```python
from build123d import *

# Parameters (mm, degrees)
SKETCH1_W           = 70
SKETCH1_H           = 70
BOSS_EXTRUDE1_DEPTH = 6
SKETCH2_R           = 20
BOSS_EXTRUDE6_DEPTH = 2.6
CUT_EXTRUDE1_START  = -2.6
CUT_EXTRUDE1_DEPTH  = 2.6
SKETCH4_R           = 3.5
CUT_EXTRUDE2_DEPTH  = 1.6
SKETCH5_R           = 1
CUT_EXTRUDE3_DEPTH  = 4.4
BOSS_EXTRUDE7_DEPTH = 2


with BuildPart() as part:
    # Sketch1 → Boss-Extrude1 (new body)
    with BuildSketch(Plane(origin=(0, 0, 0), x_dir=(1, 0, 0), z_dir=(0, 1, 0))):
        Rectangle(SKETCH1_W, SKETCH1_H)
    extrude(amount=BOSS_EXTRUDE1_DEPTH)

    # Sketch2 → Boss-Extrude6 (add)
    with BuildSketch(Plane(origin=(0, 6, 0), x_dir=(1, 0, 0), z_dir=(0, 1, 0))):
        with Locations(Location((0, 0, 0), (0, 0, 270))):
            Circle(SKETCH2_R)
        with BuildLine():
            Line((-16.28125, -2.484129312), (-0.48375, -4.272702416))
            ThreePointArc((-0.48375, -4.272702416), (0, -4.3), (0.48375, -4.272702416))
            Line((0.48375, -4.272702416), (16.28125, -2.484129312))
            ThreePointArc((16.28125, -2.484129312), (18.5, 0), (16.28125, 2.484129312))
            Line((16.28125, 2.484129312), (0.48375, 4.272702416))
            ThreePointArc((0.48375, 4.272702416), (0, 4.3), (-0.48375, 4.272702416))
            Line((-0.48375, 4.272702416), (-16.28125, 2.484129312))
            ThreePointArc((-16.28125, 2.484129312), (-18.5, 0), (-16.28125, -2.484129312))
        make_face(mode=Mode.SUBTRACT)
    extrude(amount=BOSS_EXTRUDE6_DEPTH)

    # Sketch3 → Cut-Extrude1 (cut)
    with BuildSketch(Plane(origin=(0, 6, 0), x_dir=(1, 0, 0), z_dir=(0, 1, 0)).offset(CUT_EXTRUDE1_START)):
        with BuildLine():
            Line((-4.8, 3.784022013), (-4.8, -3.784022013))
            Line((-4.8, -3.784022013), (-0.48375, -4.272702416))
            ThreePointArc((-0.48375, -4.272702416), (0, -4.3), (0.48375, -4.272702416))
            Line((0.48375, -4.272702416), (4.8, -3.784022013))
            Line((4.8, -3.784022013), (4.8, 3.784022013))
            Line((4.8, 3.784022013), (0.48375, 4.272702416))
            ThreePointArc((0.48375, 4.272702416), (0, 4.3), (-0.48375, 4.272702416))
            Line((-0.48375, 4.272702416), (-4.8, 3.784022013))
        make_face()
    extrude(amount=CUT_EXTRUDE1_DEPTH, mode=Mode.SUBTRACT)

    # Sketch4 → Cut-Extrude2 (cut)
    with BuildSketch(Plane.XZ):
        with Locations(Location((16, 0, 0), (0, 0, 90))):
            Circle(SKETCH4_R)
        with Locations(Location((-16, 0, 0), (0, 0, 270))):
            Circle(SKETCH4_R)
    extrude(amount=-CUT_EXTRUDE2_DEPTH, mode=Mode.SUBTRACT)

    # Sketch5 → Cut-Extrude3 (cut)
    with BuildSketch(Plane(origin=(0, 6, 0), x_dir=(1, 0, 0), z_dir=(0, 1, 0))):
        with Locations(Location((16, 0, 0), (0, 0, 270))):
            Circle(SKETCH5_R)
        with Locations(Location((-16, 0, 0), (0, 0, 90))):
            Circle(SKETCH5_R)
    extrude(amount=-CUT_EXTRUDE3_DEPTH, mode=Mode.SUBTRACT)

    # Sketch6 → Boss-Extrude7 (add)
    with BuildSketch(Plane(origin=(0, 8.6, 0), x_dir=(1, 0, 0), z_dir=(0, 1, 0))):
        with BuildLine():
            Line((7.187033827, 3.513765042), (0.48375, 4.272702416))
            ThreePointArc((0.48375, 4.272702416), (0, 4.3), (-0.48375, 4.272702416))
            Line((-0.48375, 4.272702416), (-7.187033827, 3.513765042))
            ThreePointArc((-7.187033827, 3.513765042), (0, 8), (7.187033827, 3.513765042))
        make_face()
        with BuildLine():
            Line((0.48375, -4.272702416), (7.187033827, -3.513765042))
            ThreePointArc((7.187033827, -3.513765042), (0, -8), (-7.187033827, -3.513765042))
            Line((-7.187033827, -3.513765042), (-0.48375, -4.272702416))
            ThreePointArc((-0.48375, -4.272702416), (0, -4.3), (0.48375, -4.272702416))
        make_face()
    extrude(amount=BOSS_EXTRUDE7_DEPTH)


solid = part.part
```
Could you check a few things on this model? Use its own coordinates, in mm. A direction names the side the tool comes from. Round coordinates to 2 decimals unless told otherwise and drop trailing zeros. Write each loop counter-clockwise with the first axis right and the second up, starting at its lowest first coordinate (ties: lowest second). Pieces come first, ordered by that corner, then holes. Notation, with made-up numbers: M 0.5,-11 L 55.5,-11 A15 cw 55.5,1 Z; hole C 78,74 d8. An arc over 180 degrees is marked long. Write each question's results on one line, items separated by ' | '. Start each with the question number.
1. I'm going to push flat-ended pins straight in: pin 1 Ø2.5 at (x, z) = (16, 0) entering from -Y; pin 2 Ø4 at (x, z) = (-9, 1.5) entering from +Y; pin 3 Ø4.5 at (x, z) = (0, -1.5) entering from +Y. Where does each tip first touch, or does it pass through?
2. On a 3-axis mill with a long thin cutter (end or side, diameter ignored), from which of +Z, -Z, +X, -X, +Y, -Y can I reach the whole of each face in a straight line? I mean faces 1 (the face through (0, 10, 8)), 2 (the face through (19.105, 0.789, 1.615)), 3 (the face through (0, 8.6, 9)), 4 (the face through (15, 4, 0)). Say none if no direction works.
3. Imagine slicing it at B-B on z = 0. Count the separate pieces of the cut face and the enclosed holes in it, and give its area (3 significant figures).
4. Thinking about a two-plate mould opening in X: for faces 5 (the face through (-18.5, 7.3, -0.1)), 6 (the face through (-35, 3, 0)), 7 (the face through (35, 3, 0)), which applies, +X half, -X half, draft (parallel to the pull), parting line (faces both ways), or undercut?
5. Imagine slicing it at D-D on z = 21.5. List the corners of the cut face in (x, y) for me, and give its area (3 significant figures).
6. Imagine slicing it at C-C on x = -6. List the corners of the cut face in (y, z) for me.
7. Imagine slicing it at A-A on y = 4.75. List the corners of the cut face in (x, z) for me.
8. I need wall thicknesses on L1, parallel to X at y = 3.05, z = 0; L2, parallel to X at y = 1.1, z = 0; L3, parallel to X at y = 5.05, z = 0. Which ranges of each line are inside material? Lowest first, please. Write a range as from..to.
Result sheet:
1) pin 1: stops at y = 1.6 | pin 2: stops at y = 8.6 | pin 3: stops at y = 3.4
2) face 1: +Z, +Y | face 2: -Y | face 3: +Y | face 4: +Y, -Y
3) separate pieces: 3 | enclosed holes: 0 | area: 363 mm^2
4) face 5: undercut | face 6: -X half | face 7: +X half
5) outline: M -35,0 L 35,0 L 35,6 L -35,6 Z | area: 420 mm^2
6) outline: M 0,-35 L 6,-35 L 6,-19.08 L 8.6,-19.08 L 8.6,-5.29 L 10.6,-5.29 L 10.6,-3.65 L 6,-3.65 L 6,3.65 L 10.6,3.65 L 10.6,5.29 L 8.6,5.29 L 8.6,19.08 L 6,19.08 L 6,35 L 0,35 Z
7) outline: M -35,-35 L 35,-35 L 35,35 L -35,35 Z; hole C -16,0 d2; hole M -4.8,-3.78 L -0.48,-4.27 A4.3 ccw 0.48,-4.27 L 4.8,-3.78 L 4.8,3.78 L 0.48,4.27 A4.3 ccw -0.48,4.27 L -4.8,3.78 Z; hole C 16,0 d2
8) L1: x = -35..-17, -15..15, 17..35 | L2: x = -35..-19.5, -12.5..12.5, 19.5..35 | L3: x = -35..-17, -15..-4.8, 4.8..15, 17..35
